```python
from build123d import *

# Parameters (mm, degrees)
SKETCH_1_W      = 87.5
SKETCH_1_H      = 99.5
SKETCH_1_R      = 1.6
EXTRUDE_1_DEPTH = 1.6
SKETCH_2_W      = 10
SKETCH_2_H      = 10
EXTRUDE_2_DEPTH = 5
SKETCH_3_W      = 25
SKETCH_3_H      = 25
EXTRUDE_3_DEPTH = 13
SKETCH_4_W      = 5
SKETCH_4_H      = 8
SKETCH_4_W_2    = 8
SKETCH_4_H_2    = 5
EXTRUDE_4_DEPTH = 7
SKETCH_5_W      = 12
SKETCH_5_H      = 7
EXTRUDE_5_DEPTH = 9
EXTRUDE_6_DEPTH = 18
SKETCH_7_R      = 2
EXTRUDE_7_DEPTH = 13
SKETCH_8_R      = 6.5
EXTRUDE_8_DEPTH = 2


with BuildPart() as part:
    # 草图1 → 凸台-拉伸1 (new body)
    with BuildSketch(Plane.XY):
        Rectangle(SKETCH_1_W, SKETCH_1_H)
        with Locations((-38.5, 45.15)):
            Circle(SKETCH_1_R, mode=Mode.SUBTRACT)
        with Locations((38.5, 45.15)):
            Circle(SKETCH_1_R, mode=Mode.SUBTRACT)
        with Locations((-38.5, -45.15)):
            Circle(SKETCH_1_R, mode=Mode.SUBTRACT)
        with Locations((38.5, -45.15)):
            Circle(SKETCH_1_R, mode=Mode.SUBTRACT)
    extrude(amount=EXTRUDE_1_DEPTH)

    # 草图2 → 凸台-拉伸2 (add)
    with BuildSketch(Plane.XY.offset(1.6)):
        with Locations((-37.75, -34.75)):
            Rectangle(SKETCH_2_W, SKETCH_2_H)
    extrude(amount=EXTRUDE_2_DEPTH)

    # 草图3 → 凸台-拉伸3 (add)
    with BuildSketch(Plane.XY.offset(1.6)):
        with Locations((3.75, -36.25)):
            Rectangle(SKETCH_3_W, SKETCH_3_H)
    extrude(amount=EXTRUDE_3_DEPTH)

    # 草图4 → 凸台-拉伸4 (add)
    with BuildSketch(Plane.XY.offset(1.6)):
        with Locations((-31.25, 44.75)):
            Rectangle(SKETCH_4_W, SKETCH_4_H)
        with Locations((-25.25, 44.75)):
            Rectangle(SKETCH_4_W, SKETCH_4_H)
        with Locations((-19.25, 44.75)):
            Rectangle(SKETCH_4_W, SKETCH_4_H)
        with Locations((-13.25, 44.75)):
            Rectangle(SKETCH_4_W, SKETCH_4_H)
        with Locations((-7.25, 44.75)):
            Rectangle(SKETCH_4_W, SKETCH_4_H)
        with Locations((-1.25, 44.75)):
            Rectangle(SKETCH_4_W, SKETCH_4_H)
        with Locations((4.75, 44.75)):
            Rectangle(SKETCH_4_W, SKETCH_4_H)
        with Locations((10.75, 44.75)):
            Rectangle(SKETCH_4_W, SKETCH_4_H)
        with Locations((16.75, 44.75)):
            Rectangle(SKETCH_4_W, SKETCH_4_H)
        with Locations((22.75, 44.75)):
            Rectangle(SKETCH_4_W, SKETCH_4_H)
        with Locations((-38.75, -24.25)):
            Rectangle(SKETCH_4_W_2, SKETCH_4_H_2)
        with Locations((-38.75, -18.25)):
            Rectangle(SKETCH_4_W_2, SKETCH_4_H_2)
        with Locations((-38.75, -12.25)):
            Rectangle(SKETCH_4_W_2, SKETCH_4_H_2)
        with Locations((-38.75, -6.25)):
            Rectangle(SKETCH_4_W_2, SKETCH_4_H_2)
        with Locations((-38.75, -0.25)):
            Rectangle(SKETCH_4_W_2, SKETCH_4_H_2)
        with Locations((-38.75, 5.75)):
            Rectangle(SKETCH_4_W_2, SKETCH_4_H_2)
        with Locations((-38.75, 11.75)):
            Rectangle(SKETCH_4_W_2, SKETCH_4_H_2)
        with Locations((-38.75, 17.75)):
            Rectangle(SKETCH_4_W_2, SKETCH_4_H_2)
        with Locations((38.75, -37.25)):
            Rectangle(SKETCH_4_W_2, SKETCH_4_H_2)
        with Locations((38.75, -31.25)):
            Rectangle(SKETCH_4_W_2, SKETCH_4_H_2)
        with Locations((38.75, -25.25)):
            Rectangle(SKETCH_4_W_2, SKETCH_4_H_2)
        with Locations((38.75, -19.25)):
            Rectangle(SKETCH_4_W_2, SKETCH_4_H_2)
        with Locations((38.75, -13.25)):
            Rectangle(SKETCH_4_W_2, SKETCH_4_H_2)
        with Locations((38.75, -7.25)):
            Rectangle(SKETCH_4_W_2, SKETCH_4_H_2)
        with Locations((38.75, -1.25)):
            Rectangle(SKETCH_4_W_2, SKETCH_4_H_2)
        with Locations((38.75, 4.75)):
            Rectangle(SKETCH_4_W_2, SKETCH_4_H_2)
        with Locations((-6.75, -19.25)):
            Rectangle(SKETCH_4_W_2, SKETCH_4_H_2)
    extrude(amount=EXTRUDE_4_DEPTH)

    # 草图5 → 凸台-拉伸5 (add)
    with BuildSketch(Plane.XY.offset(1.6)):
        with Locations((36.75, 11.25)):
            Rectangle(SKETCH_5_W, SKETCH_5_H)
        with Locations((36.75, 21.25)):
            Rectangle(SKETCH_5_W, SKETCH_5_H)
    extrude(amount=EXTRUDE_5_DEPTH)

    # 草图6 → 凸台-拉伸6 (add)
    with BuildSketch(Plane.XY.offset(1.6)):
        with BuildLine():
            Line((-20.75, -36.75), (-12.75, -36.75))
            ThreePointArc((-12.75, -36.75), (-9.75, -39.75), (-12.75, -42.75))
            Line((-12.75, -42.75), (-20.75, -42.75))
            ThreePointArc((-20.75, -42.75), (-23.75, -39.75), (-20.75, -36.75))
        make_face()
    extrude(amount=EXTRUDE_6_DEPTH)

    # 草图7 → 凸台-拉伸7 (add)
    with BuildSketch(Plane.XY.offset(1.6)):
        with Locations(Location((-20.75, -31.75, 0), (0, 0, 180))):
            Circle(SKETCH_7_R)
        with Locations(Location((-15.75, -31.75, 0), (0, 0, 180))):
            Circle(SKETCH_7_R)
        with Locations(Location((19.75, -41.25, 0), (0, 0, 180))):
            Circle(SKETCH_7_R)
        with Locations(Location((19.75, -46.25, 0), (0, 0, 180))):
            Circle(SKETCH_7_R)
    extrude(amount=EXTRUDE_7_DEPTH)

    # 草图8 → 凸台-拉伸8 (add)
    with BuildSketch(Plane(origin=(0, -47.75, 0), x_dir=(-1, 0, 0), z_dir=(0, -1, 0))):
        with Locations((17, -7.6)):
            Circle(SKETCH_8_R)
    extrude(amount=-EXTRUDE_8_DEPTH)


solid = part.part
```
Read the model definition and answer for the solid it produces. Units are mm, in the model's axes. A direction names the side the tool comes from. Give positions to 0.01 mm unless a question says otherwise; leave off trailing zeros. Write each loop counter-clockwise with the first axis right and the second up, starting at its lowest first coordinate (ties: lowest second). Pieces come first, ordered by that corner, then holes. Notation, with made-up numbers: (2, 42.5) -> (35, 42.5) arc R18 cw to (35, 63.5) -> close; hole circle Ø3 at (6, -34). An arc over 180 degrees is marked (long way). Answer in a Markdown table with one row per item.
1) Section D-D on z = 17.25 is taken. Give the vertices of the cut face in (x, y), plus the area to 3 significant figures.
Results list:
| item | result |
|---|---|
| outline | (-20.75, -42.75) -> (-12.75, -42.75) arc R3 ccw to (-12.75, -36.75) -> (-20.75, -36.75) arc R3 ccw to start |
| area | 76.3 mm^2 |
2) Section A-A on y = 4.5 is taken. Give the vertices of the cut face in (x, z).
Results list:
| item | result |
|---|---|
| outline | (-43.75, 0) -> (43.75, 0) -> (43.75, 1.6) -> (42.75, 1.6) -> (42.75, 8.6) -> (34.75, 8.6) -> (34.75, 1.6) -> (-34.75, 1.6) -> (-34.75, 8.6) -> (-42.75, 8.6) -> (-42.75, 1.6) -> (-43.75, 1.6) -> close |
3) A tool of negligible diameter and unlimited length cuts with its end or side. For faces 1 (the flat face through (42.75, 21, 6)), 2 (the flat face through (-32.75, -35, 4)), 3 (the flat face through (-7, -19, 8.6)), from which of +Z, -Z, +X, -X, +Y, -Y can it reach the whole face along a straight path? Write none if from no direction.
Results list:
| item | result |
|---|---|
| face 1 | +Z, +X, +Y, -Y |
| face 2 | +Z, -Y |
| face 3 | +Z, +X, -X, +Y |
4) Determine the mould class of faces 4 (the flat face through (-31, 40.75, 5)), 5 (the flat face through (2.25, 45, 5)), 6 (the flat face through (-31, 48.75, 5)) for opening direction Y: released by +Y, released by -Y, zero draft, split by the parting line, or undercut.
Results list:
| item | result |
|---|---|
| face 4 | undercut |
| face 5 | zero draft |
| face 6 | released by +Y |
5) Straight lines are drawn through the part: line 1 (Y direction, x = 38.5, z = 0.55); line 2 (Y direction, x = 33, z = 9.75); line 3 (X direction, y = -43.5, z = 9.75). For each, find the intervals that lie inside material, in ascending order. Write a range as [from, to].
Results list:
| item | result |
|---|---|
| line 1 | [-49.75, -46.75], [-43.55, 43.55], [46.75, 49.75] |
| line 2 | [7.75, 14.75], [17.75, 24.75] |
| line 3 | [-8.75, 16.25] |
6) Section B-B on z = 12.5 is taken. Give the vertices of the cut face in (x, y), plus the area to 3 significant figures.
Results list:
| item | result |
|---|---|
| outline | circle Ø4 at (-20.75, -31.75); (-21.27, -47.75) -> (-12.73, -47.75) -> (-12.73, -45.75) -> (-21.27, -45.75) -> close; (-20.75, -42.75) -> (-12.75, -42.75) arc R3 ccw to (-12.75, -36.75) -> (-20.75, -36.75) arc R3 ccw to start; circle Ø4 at (-15.75, -31.75); (-8.75, -48.75) -> (16.25, -48.75) -> (16.25, -23.75) -> (-8.75, -23.75) -> close; circle Ø4 at (19.75, -46.25); circle Ø4 at (19.75, -41.25) |
| area | 769 mm^2 |
7) Section C-C on x = -38.5 is taken. Count the separate pieces of the cut face and the enclosed holes in it, plus the area to 3 significant figures.
Results list:
| item | result |
|---|---|
| separate pieces | 3 |
| enclosed holes | 0 |
| area | 479 mm^2 |
8) Each of these flat-tipped pins is pushed along its axis until it touches: pin 1 Ø4 at (x, z) = (4, 4.5) entering from -Y; pin 2 Ø5.5 at (x, y) = (-13.5, 44.5) entering from +Z; pin 3 Ø5.5 at (y, z) = (45.5, 5) entering from -X; pin 4 Ø7.5 at (y, z) = (46, 4) entering from +X. Where does it stop, or does it pass through?
Results list:
| item | result |
|---|---|
| pin 1 | y = -48.75 |
| pin 2 | z = 8.6 |
| pin 3 | x = -33.75 |
| pin 4 | x = 43.75 |
